Work out the finished part from the listing and answer in its coordinate system (mm). A direction names the side the tool comes from. Give positions to 0.01 mm unless a question says otherwise; leave off trailing zeros. Order: outer loops, then holes, each group sorted by start corner. A loop starts at its lowest first (then second) coordinate and runs counter-clockwise, first axis right, second up. Notation, with made-up numbers: M 50.5,7.25 L 104.5,7.25 A28 cw 104.5,30.25 Z; hole C -22.75,82 d5. An arc over 180 degrees is marked long. One line per item, written item: value.
from build123d import *

# Parameters (mm, degrees)
BOSS_EXTRUDE1_DEPTH = 10
CUT_EXTRUDE1_DEPTH  = 3
SKETCH3_R           = 6
CUT_EXTRUDE2_DEPTH  = 5
SKETCH3_3_R         = 3
CUT_EXTRUDE3_DEPTH  = 179.204938203
CIRPATTERN1_COUNT   = 6
SKETCH4_R           = 12.5
CUT_EXTRUDE4_DEPTH  = 10
SKETCH4_3_R         = 8
CUT_EXTRUDE5_DEPTH  = 179.204938203
SKETCH5_R           = 5
CUT_EXTRUDE6_DEPTH  = 15


with BuildPart() as part:
    # Sketch1 → Boss-Extrude1 (new, symmetric)
    with BuildSketch(Plane(origin=(0, 0, 0), x_dir=(0, 0, -1), z_dir=(1, 0, 0))):
        with BuildLine():
            Line((46, 125), (46, 0))
            Line((46, 0), (-46, 0))
            Line((-46, 0), (-46, 125))
            ThreePointArc((-46, 125), (0, 171), (46, 125))
        make_face()
    extrude(amount=BOSS_EXTRUDE1_DEPTH, both=True)

    # Sketch2 → Cut-Extrude1 (cut)
    with BuildSketch(Plane(origin=(10, 0, 0), x_dir=(0, 0, -1), z_dir=(1, 0, 0))):
        with BuildLine():
            Line((-34, 74.206299603), (-34, 18))
            ThreePointArc((-34, 18), (-32.242640687, 13.757359313), (-28, 12))
            Line((-28, 12), (28, 12))
            ThreePointArc((28, 12), (32.242640687, 13.757359313), (34, 18))
            Line((34, 18), (34, 74.206299603))
            ThreePointArc((34, 74.206299603), (31.051285766, 79.372502771), (25.103448276, 79.460820334))
            ThreePointArc((25.103448276, 79.460820334), (0, 73), (-25.103448276, 79.460820334))
            ThreePointArc((-25.103448276, 79.460820334), (-31.051285766, 79.372502771), (-34, 74.206299603))
        make_face()
    cut_extrude1 = extrude(amount=-CUT_EXTRUDE1_DEPTH, mode=Mode.SUBTRACT)

    # Mirror1: Cut-Extrude1 across plane
    add(cut_extrude1.mirror(Plane(origin=(0, 0, 0), x_dir=(0, 0, 1), z_dir=(1, 0, 0))), mode=Mode.SUBTRACT)

    # Sketch3 → Cut-Extrude2 (cut)
    with BuildSketch(Plane(origin=(10, 0, 0), x_dir=(0, 0, -1), z_dir=(1, 0, 0))):
        with Locations((0, 164)):
            Circle(SKETCH3_R)
    cut_extrude2 = extrude(amount=-CUT_EXTRUDE2_DEPTH, mode=Mode.SUBTRACT)

    # Sketch3_3 → Cut-Extrude3 (cut, through all)
    with BuildSketch(Plane(origin=(10, 0, 0), x_dir=(0, 0, -1), z_dir=(1, 0, 0))):
        with Locations((0, 164)):
            Circle(SKETCH3_3_R)
    cut_extrude3 = extrude(amount=-CUT_EXTRUDE3_DEPTH, mode=Mode.SUBTRACT)

    # CirPattern1: Cut-Extrude2, Cut-Extrude3 ×6 about axis
    cirpattern1_axis = Axis((0, 125, 0), (1, 0, 0))
    add([cut_extrude2.rotate(cirpattern1_axis, i * 360 / CIRPATTERN1_COUNT) for i in range(1, CIRPATTERN1_COUNT)], mode=Mode.SUBTRACT)
    add([cut_extrude3.rotate(cirpattern1_axis, i * 360 / CIRPATTERN1_COUNT) for i in range(1, CIRPATTERN1_COUNT)], mode=Mode.SUBTRACT)

    # Sketch4 → Cut-Extrude4 (cut)
    with BuildSketch(Plane(origin=(10, 0, 0), x_dir=(0, 0, -1), z_dir=(1, 0, 0))):
        with Locations((0, 125)):
            Circle(SKETCH4_R)
    extrude(amount=-CUT_EXTRUDE4_DEPTH, mode=Mode.SUBTRACT)

    # Sketch4_3 → Cut-Extrude5 (cut, through all)
    with BuildSketch(Plane(origin=(10, 0, 0), x_dir=(0, 0, -1), z_dir=(1, 0, 0))):
        with Locations((0, 125)):
            Circle(SKETCH4_3_R)
    extrude(amount=-CUT_EXTRUDE5_DEPTH, mode=Mode.SUBTRACT)

    # Sketch5 → Cut-Extrude6 (cut)
    with BuildSketch(Plane.XZ):
        with Locations(Location((0, 30, 0), (0, 0, 270))):
            Circle(SKETCH5_R)
        with Locations(Location((0, -30, 0), (0, 0, 270))):
            Circle(SKETCH5_R)
    extrude(amount=-CUT_EXTRUDE6_DEPTH, mode=Mode.SUBTRACT)


solid = part.part
(1) Determine the mould class of faces 6 (the flat face through (10, 87, -11)), 7 (the cylindrical face through (-8.521, 13.711, -32.196)) for opening direction Z: pulls with the +Z half, pulls with the -Z half, needs draft (parallel to the pull), parting line crosses it, or undercut.
Findings:
face 6: needs draft
face 7: undercut
(2) Section D-D, the plane z = 22 is taken. Give the vertices of the cut face in (x, y).
Findings:
outline: M -10,0 L 10,0 L 10,12 L 7,12 L 7,77.88 L 10,77.88 L 10,165.4 L -10,165.4 L -10,77.88 L -7,77.88 L -7,12 L -10,12 Z
(3) Section C-C, the plane x = 2 is taken. Give the vertices of the cut face in (y, z) (3 decimals).
Findings:
outline: M 0,-46 L 125,-46 A46 ccw 125,46 L 0,46 L 0,34.583 L 15,34.583 L 15,25.417 L 0,25.417 L 0,-25.417 L 15,-25.417 L 15,-34.583 L 0,-34.583 Z; hole C 86,0 d6; hole C 105.5,-33.775 d6; hole C 105.5,33.775 d6; hole C 125,0 d25; hole C 144.5,-33.775 d6; hole C 144.5,33.775 d6; hole C 164,0 d6
(4) Section A-A, the plane y = 105.5 is taken. Give the vertices of the cut face in (x, z) (3 decimals), then the cut area to 3 significant figures.
Findings:
outline: M -10,-46 L 10,-46 L 10,-39.775 L 5,-39.775 L 5,-36.775 L -10,-36.775 Z; M -10,-30.775 L 5,-30.775 L 5,-27.775 L 10,-27.775 L 10,27.775 L 5,27.775 L 5,30.775 L -10,30.775 Z; M -10,36.775 L 5,36.775 L 5,39.775 L 10,39.775 L 10,46 L -10,46 Z
area: 1,540 mm^2
(5) Which of the six approach directions +Z, -Z, +X, -X, +Y, -Y give full straight-line access (tool end or side, diameter ignored) to faces 1 (the flat face through (5, 87, -3)), 2 (the cylindrical face through (0, 7, -25)), 3 (the flat face through (-7, 47, 0)), 4 (the flat face through (-10, 87, 10)), 5 (the cylindrical face through (-2.395, 141.526, -34.166))?
Findings:
face 1: +X
face 2: -Y
face 3: -X
face 4: +Z, -Z, -X, +Y, -Y
face 5: +X, -X
(6) Section B-B, the plane y = 86 is taken. Give the vertices of the cut face in (x, z), then the cut area to 3 significant figures.
Findings:
outline: M -10,-46 L 10,-46 L 10,-6 L 5,-6 L 5,-3 L -10,-3 Z; M -10,3 L 5,3 L 5,6 L 10,6 L 10,46 L -10,46 Z
area: 1,690 mm^2
(7) Given P1, Ø7, axis at y = 105.5, z = -33.77, coming from the -X side; P2, Ø5.5, axis at y = 144.5, z = 33.77, coming from the +X side; P3, Ø10, axis at x = -3, z = -6, coming from the +Y side; P4, Ø4, axis at x = -3.5, z = 35, coming from the +Y side, each flat-ended and moving along its own axis, determine where each tip first touches the part or whether it passes through.
Findings:
P1: stops at x = -10
P2: passes through
P3: stops at y = 170.99
P4: stops at y = 157.05
(8) Find the intervals of material crossed by probe 1 along Y at (x, z) = (-2.5, 0); probe 2 along Y at (x, z) = (8, 31); probe 3 along Z at (x, y) = (2.75, 147), in increasing order. Write a range as from..to.
Findings:
probe 1: y = 0..83, 89..117, 133..161, 167..171
probe 2: y = 0..12.8, 79.4..100.18, 110.82..139.18, 149.82..158.99
probe 3: z = -40.4..-35.43, -32.12..32.12, 35.43..40.4
